from build123d import *

# Parameters (mm, degrees)
SKETCH1_W           = 88
SKETCH1_H           = 40
BOSS_EXTRUDE1_DEPTH = 3.175
CUT_EXTRUDE1_REACH  = 5.175
SKETCH2_W           = 16
SKETCH2_H           = 3.175
SKETCH2_W_2         = 8
CUT_EXTRUDE2_REACH  = 5.175
SKETCH3_W           = 3.175
SKETCH3_H           = 8
CUT_EXTRUDE3_REACH  = 5.175
SKETCH4_R           = 7


with BuildPart() as part:
    # Sketch1 → Boss-Extrude1 (new body)
    with BuildSketch(Plane(origin=(0, 0, 0), x_dir=(1, 0, 0), z_dir=(0, 1, 0))):
        with Locations((44, -20)):
            Rectangle(SKETCH1_W, SKETCH1_H)
    extrude(amount=BOSS_EXTRUDE1_DEPTH)

    # Sketch2 → Cut-Extrude1 (cut, up to next)
    with BuildSketch(Plane(origin=(0, 3.175, 0), x_dir=(1, 0, 0), z_dir=(0, 1, 0)), mode=Mode.PRIVATE) as cut_extrude1_sk1:
        with Locations((8, -1.5875)):
            Rectangle(SKETCH2_W, SKETCH2_H)
    cut_extrude1_tool1 = extrude(cut_extrude1_sk1.sketch, amount=-CUT_EXTRUDE1_REACH, mode=Mode.PRIVATE) & part.part
    add(cut_extrude1_tool1.solids().sort_by_distance((8, 3.175, 1.5875))[0], mode=Mode.SUBTRACT)
    # Sketch2 → Cut-Extrude1 (cut, up to next)
    with BuildSketch(Plane(origin=(0, 3.175, 0), x_dir=(1, 0, 0), z_dir=(0, 1, 0)), mode=Mode.PRIVATE) as cut_extrude1_sk2:
        with Locations((44, -1.5875)):
            Rectangle(SKETCH2_W_2, SKETCH2_H)
    cut_extrude1_tool2 = extrude(cut_extrude1_sk2.sketch, amount=-CUT_EXTRUDE1_REACH, mode=Mode.PRIVATE) & part.part
    add(cut_extrude1_tool2.solids().sort_by_distance((44, 3.175, 1.5875))[0], mode=Mode.SUBTRACT)
    # Sketch2 → Cut-Extrude1 (cut, up to next)
    with BuildSketch(Plane(origin=(0, 3.175, 0), x_dir=(1, 0, 0), z_dir=(0, 1, 0)), mode=Mode.PRIVATE) as cut_extrude1_sk3:
        with Locations((60, -1.5875)):
            Rectangle(SKETCH2_W_2, SKETCH2_H)
    cut_extrude1_tool3 = extrude(cut_extrude1_sk3.sketch, amount=-CUT_EXTRUDE1_REACH, mode=Mode.PRIVATE) & part.part
    add(cut_extrude1_tool3.solids().sort_by_distance((60, 3.175, 1.5875))[0], mode=Mode.SUBTRACT)
    # Sketch2 → Cut-Extrude1 (cut, up to next)
    with BuildSketch(Plane(origin=(0, 3.175, 0), x_dir=(1, 0, 0), z_dir=(0, 1, 0)), mode=Mode.PRIVATE) as cut_extrude1_sk4:
        with Locations((80, -1.5875)):
            Rectangle(SKETCH2_W, SKETCH2_H)
    cut_extrude1_tool4 = extrude(cut_extrude1_sk4.sketch, amount=-CUT_EXTRUDE1_REACH, mode=Mode.PRIVATE) & part.part
    add(cut_extrude1_tool4.solids().sort_by_distance((80, 3.175, 1.5875))[0], mode=Mode.SUBTRACT)
    # Sketch2 → Cut-Extrude1 (cut, up to next)
    with BuildSketch(Plane(origin=(0, 3.175, 0), x_dir=(1, 0, 0), z_dir=(0, 1, 0)), mode=Mode.PRIVATE) as cut_extrude1_sk5:
        with Locations((28, -1.5875)):
            Rectangle(SKETCH2_W_2, SKETCH2_H)
    cut_extrude1_tool5 = extrude(cut_extrude1_sk5.sketch, amount=-CUT_EXTRUDE1_REACH, mode=Mode.PRIVATE) & part.part
    add(cut_extrude1_tool5.solids().sort_by_distance((28, 3.175, 1.5875))[0], mode=Mode.SUBTRACT)
    # Sketch2 → Cut-Extrude1 (cut, up to next)
    with BuildSketch(Plane(origin=(0, 3.175, 0), x_dir=(1, 0, 0), z_dir=(0, 1, 0)), mode=Mode.PRIVATE) as cut_extrude1_sk6:
        with Locations((44, -38.4125)):
            Rectangle(SKETCH2_W_2, SKETCH2_H)
    cut_extrude1_tool6 = extrude(cut_extrude1_sk6.sketch, amount=-CUT_EXTRUDE1_REACH, mode=Mode.PRIVATE) & part.part
    add(cut_extrude1_tool6.solids().sort_by_distance((44, 3.175, 38.4125))[0], mode=Mode.SUBTRACT)
    # Sketch2 → Cut-Extrude1 (cut, up to next)
    with BuildSketch(Plane(origin=(0, 3.175, 0), x_dir=(1, 0, 0), z_dir=(0, 1, 0)), mode=Mode.PRIVATE) as cut_extrude1_sk7:
        with Locations((28, -38.4125)):
            Rectangle(SKETCH2_W_2, SKETCH2_H)
    cut_extrude1_tool7 = extrude(cut_extrude1_sk7.sketch, amount=-CUT_EXTRUDE1_REACH, mode=Mode.PRIVATE) & part.part
    add(cut_extrude1_tool7.solids().sort_by_distance((28, 3.175, 38.4125))[0], mode=Mode.SUBTRACT)
    # Sketch2 → Cut-Extrude1 (cut, up to next)
    with BuildSketch(Plane(origin=(0, 3.175, 0), x_dir=(1, 0, 0), z_dir=(0, 1, 0)), mode=Mode.PRIVATE) as cut_extrude1_sk8:
        with Locations((8, -38.4125)):
            Rectangle(SKETCH2_W, SKETCH2_H)
    cut_extrude1_tool8 = extrude(cut_extrude1_sk8.sketch, amount=-CUT_EXTRUDE1_REACH, mode=Mode.PRIVATE) & part.part
    add(cut_extrude1_tool8.solids().sort_by_distance((8, 3.175, 38.4125))[0], mode=Mode.SUBTRACT)
    # Sketch2 → Cut-Extrude1 (cut, up to next)
    with BuildSketch(Plane(origin=(0, 3.175, 0), x_dir=(1, 0, 0), z_dir=(0, 1, 0)), mode=Mode.PRIVATE) as cut_extrude1_sk9:
        with Locations((80, -38.4125)):
            Rectangle(SKETCH2_W, SKETCH2_H)
    cut_extrude1_tool9 = extrude(cut_extrude1_sk9.sketch, amount=-CUT_EXTRUDE1_REACH, mode=Mode.PRIVATE) & part.part
    add(cut_extrude1_tool9.solids().sort_by_distance((80, 3.175, 38.4125))[0], mode=Mode.SUBTRACT)
    # Sketch2 → Cut-Extrude1 (cut, up to next)
    with BuildSketch(Plane(origin=(0, 3.175, 0), x_dir=(1, 0, 0), z_dir=(0, 1, 0)), mode=Mode.PRIVATE) as cut_extrude1_sk10:
        with Locations((60, -38.4125)):
            Rectangle(SKETCH2_W_2, SKETCH2_H)
    cut_extrude1_tool10 = extrude(cut_extrude1_sk10.sketch, amount=-CUT_EXTRUDE1_REACH, mode=Mode.PRIVATE) & part.part
    add(cut_extrude1_tool10.solids().sort_by_distance((60, 3.175, 38.4125))[0], mode=Mode.SUBTRACT)

    # Sketch3 → Cut-Extrude2 (cut, up to next)
    with BuildSketch(Plane(origin=(0, 3.175, 0), x_dir=(1, 0, 0), z_dir=(0, 1, 0)), mode=Mode.PRIVATE) as cut_extrude2_sk1:
        with Locations((1.5875, -28)):
            Rectangle(SKETCH3_W, SKETCH3_H)
    cut_extrude2_tool1 = extrude(cut_extrude2_sk1.sketch, amount=-CUT_EXTRUDE2_REACH, mode=Mode.PRIVATE) & part.part
    add(cut_extrude2_tool1.solids().sort_by_distance((1.5875, 3.175, 28))[0], mode=Mode.SUBTRACT)
    # Sketch3 → Cut-Extrude2 (cut, up to next)
    with BuildSketch(Plane(origin=(0, 3.175, 0), x_dir=(1, 0, 0), z_dir=(0, 1, 0)), mode=Mode.PRIVATE) as cut_extrude2_sk2:
        with Locations((1.5875, -12)):
            Rectangle(SKETCH3_W, SKETCH3_H)
    cut_extrude2_tool2 = extrude(cut_extrude2_sk2.sketch, amount=-CUT_EXTRUDE2_REACH, mode=Mode.PRIVATE) & part.part
    add(cut_extrude2_tool2.solids().sort_by_distance((1.5875, 3.175, 12))[0], mode=Mode.SUBTRACT)
    # Sketch3 → Cut-Extrude2 (cut, up to next)
    with BuildSketch(Plane(origin=(0, 3.175, 0), x_dir=(1, 0, 0), z_dir=(0, 1, 0)), mode=Mode.PRIVATE) as cut_extrude2_sk3:
        with Locations((86.4125, -28)):
            Rectangle(SKETCH3_W, SKETCH3_H)
    cut_extrude2_tool3 = extrude(cut_extrude2_sk3.sketch, amount=-CUT_EXTRUDE2_REACH, mode=Mode.PRIVATE) & part.part
    add(cut_extrude2_tool3.solids().sort_by_distance((86.4125, 3.175, 28))[0], mode=Mode.SUBTRACT)
    # Sketch3 → Cut-Extrude2 (cut, up to next)
    with BuildSketch(Plane(origin=(0, 3.175, 0), x_dir=(1, 0, 0), z_dir=(0, 1, 0)), mode=Mode.PRIVATE) as cut_extrude2_sk4:
        with Locations((86.4125, -12)):
            Rectangle(SKETCH3_W, SKETCH3_H)
    cut_extrude2_tool4 = extrude(cut_extrude2_sk4.sketch, amount=-CUT_EXTRUDE2_REACH, mode=Mode.PRIVATE) & part.part
    add(cut_extrude2_tool4.solids().sort_by_distance((86.4125, 3.175, 12))[0], mode=Mode.SUBTRACT)

    # Sketch4 → Cut-Extrude3 (cut, up to next)
    with BuildSketch(Plane(origin=(0, 3.175, 0), x_dir=(1, 0, 0), z_dir=(0, 1, 0)), mode=Mode.PRIVATE) as cut_extrude3_sk1:
        with Locations((13.25, -26.915)):
            Circle(SKETCH4_R)
    cut_extrude3_tool1 = extrude(cut_extrude3_sk1.sketch, amount=-CUT_EXTRUDE3_REACH, mode=Mode.PRIVATE) & part.part
    add(cut_extrude3_tool1.solids().sort_by_distance((13.25, 3.175, 26.915))[0], mode=Mode.SUBTRACT)
    # Sketch4 → Cut-Extrude3 (cut, up to next)
    with BuildSketch(Plane(origin=(0, 3.175, 0), x_dir=(1, 0, 0), z_dir=(0, 1, 0)), mode=Mode.PRIVATE) as cut_extrude3_sk2:
        with Locations((48.25, -26.915)):
            Circle(SKETCH4_R)
    cut_extrude3_tool2 = extrude(cut_extrude3_sk2.sketch, amount=-CUT_EXTRUDE3_REACH, mode=Mode.PRIVATE) & part.part
    add(cut_extrude3_tool2.solids().sort_by_distance((48.25, 3.175, 26.915))[0], mode=Mode.SUBTRACT)


solid = part.part
Design review of the part built by this model. Coordinates are the model's own, in mm. A direction names the side the tool comes from. Coordinates: 2 decimals unless noted, no trailing zeros. Order: outer loops, then holes, each group sorted by start corner. A loop starts at its lowest first (then second) coordinate and runs counter-clockwise, first axis right, second up.
Item 1: Take a section at B-B, the plane z = 29. Write out the cut boundary in (x, y) (3 decimals).
Item 2: Take a section at D-D, the plane x = 60.5. Write out the cut boundary in (y, z) (3 decimals).
Item 3: For line 1 (X direction, y = 2.1, z = 37); line 2 (Z direction, x = 13.25, y = 2.5) (3 decimals); line 3 (X direction, y = 1.85, z = 29) (3 decimals), list the stretches that pass through material, from the lowest coordinate up.
Item 4: Take a section at A-A, the plane x = 13.25. Write out the cut boundary in (y, z) (3 decimals).
Item 5: The part is to be moulded in two halves that separate along Z. For faces 1 (the flat face through (2, 2, 24)), 2 (the flat face through (52, 2, 0)), 3 (the flat face through (40, 2, 2)), 4 (the flat face through (3.175, 2, 12)), say which applies: pulls with the +Z half, pulls with the -Z half, needs draft (parallel to the pull), parting line crosses it, or undercut.
Item 6: For faces 5 (the flat face through (28, 2, 36.825)), 6 (the flat face through (3.175, 2, 28)), 7 (the flat face through (84.825, 2, 12)), 8 (the flat face through (24, 2, 2)), list the 3-axis set-ups (+Z, -Z, +X, -X, +Y, -Y) from which the entire face can be reached by the end or side of a thin tool; tool diameter is ignored.
Item 7: Take a section at C-C, the plane x = 42.5. Write out the cut boundary in (y, z) (3 decimals).
Item 8: For pin 1 Ø1 at (y, z) = (2.5, 2) entering from +X; pin 2 Ø1 at (y, z) = (2, 37.5) entering from -X; pin 3 Ø1.6 at (x, y) = (58.5, 2) entering from +Z (3 decimals), all flat-tipped, find the tip position at first contact; note any pin that passes through.
The answers:
1. outline: (3.175, 0) - (6.568, 0) - (6.568, 3.175) - (3.175, 3.175) - close; (19.932, 0) - (41.568, 0) - (41.568, 3.175) - (19.932, 3.175) - close; (54.932, 0) - (84.825, 0) - (84.825, 3.175) - (54.932, 3.175) - close
2. outline: (0, 3.175) - (3.175, 3.175) - (3.175, 36.825) - (0, 36.825) - close
3. line 1: x = 16 to 24, 32 to 40, 48 to 56, 64 to 72
3. line 2: z = 3.175 to 19.915, 33.915 to 36.825
3. line 3: x = 3.175 to 6.568, 19.932 to 41.568, 54.932 to 84.825
4. outline: (0, 3.175) - (3.175, 3.175) - (3.175, 19.915) - (0, 19.915) - close; (0, 33.915) - (3.175, 33.915) - (3.175, 36.825) - (0, 36.825) - close
5. face 1: undercut
5. face 2: pulls with the -Z half
5. face 3: needs draft
5. face 4: undercut
6. face 5: +Z, +Y, -Y
6. face 6: -X, +Y, -Y
6. face 7: +X, +Y, -Y
6. face 8: -Z, +Y, -Y
7. outline: (0, 3.175) - (3.175, 3.175) - (3.175, 22.923) - (0, 22.923) - close; (0, 30.907) - (3.175, 30.907) - (3.175, 36.825) - (0, 36.825) - close
8. pin 1: stops at x = 72
8. pin 2: stops at x = 16
8. pin 3: stops at z = 36.825
